Model file for the job. Use its own axes, mm. Round coordinates to 2 decimals unless told otherwise and drop trailing zeros. Order: outer loops, then holes, each group sorted by start corner. A loop starts at its lowest first (then second) coordinate and runs counter-clockwise, first axis right, second up. Notation, with made-up numbers: (-9.5, -19) - (-5.5, -19) arc R22 ccw to (-5.5, -11) - close; hole circle Ø3 at (45.5, 11). An arc over 180 degrees is marked (long way). Put each result on its own line as item: value. Start each with the question number.
Item 1: Mould opens along Z. For faces 1 (the face through (-0.29, 1.68, -1.32)), 2 (the face through (-2, 0, 0)), 3 (the face through (0.867, 0.197, 3.905)) say: pulls with the +Z half, pulls with the -Z half, needs draft (parallel to the pull), parting line crosses it, or undercut.
Item 2: Saw through at B-B on x = 0. List the corners of the cut face in (y, z), plus the area to 3 significant figures.
Item 3: Probe probe 1 along Z at (x, y) = (0, 2.5); probe 2 along Y at (x, z) = (3.25, -1.75); probe 3 along Z at (x, y) = (-1, 2.9). List the from-to ranges inside material, lowest first.
Item 4: Saw through at D-D on x = 1.75. List the corners of the cut face in (y, z).
Item 5: Saw through at C-C on z = -2.5. List the corners of the cut face in (x, y).
Item 6: Saw through at A-A on z = 0. List the corners of the cut face in (x, y).
Item 7: Pin check, flat tips, straight feed: pin 1 Ø2 at (x, y) = (-2, 1) entering from -Z; pin 2 Ø2 at (x, y) = (-2, 0.5) entering from -Z; pin 3 Ø1.5 at (x, y) = (3, 3) entering from +Z. Stop position of each tip, or through.
Autodesk Inventor part; units mm, degrees
ref_plane "YZ Plane" through (0, 0, 0) normal (1, 0, 0) x (0, 1, 0)
ref_plane "XZ Plane" through (0, 0, 0) normal (0, 1, 0) x (-1, 0, 0)
ref_plane "XY Plane" through (0, 0, 0) normal (0, 0, 1) x (1, 0, 0)
sketch "スケッチ1" plane through (0, 0, 0) normal (0, 1, 0) x (-1, 0, 0)
  circle A0 centre (0, 0) radius 4
  dimension "d0" = 8
extrude "押し出し1" add sketch "スケッチ1" along normal blind 0.4
sketch "スケッチ2" plane through (0, 0.4, 0) normal (0, 1, 0) x (1, 0, 0)
  circle A0 centre (0, 0) radius 3
  dimension "d3" = 6
extrude "押し出し2" add sketch "スケッチ2" along normal blind 3
sketch "スケッチ3" plane through (0, 0, 0) normal (0, -1, 0) x (1, 0, 0)
  circle A0 centre (0, 0) radius 1.35
  dimension "d6" = 2.7
extrude "押し出し3" cut sketch "スケッチ3" against normal through all
properties part number "screw_bearing_setter"
Results found:
1. face 1: undercut
1. face 2: needs draft
1. face 3: parting line crosses it
2. outline: (0, -4) - (0.4, -4) - (0.4, -3) - (3.4, -3) - (3.4, -1.35) - (0, -1.35) - close; (0, 1.35) - (3.4, 1.35) - (3.4, 3) - (0.4, 3) - (0.4, 4) - (0, 4) - close
2. area: 12.0 mm²
3. probe 1: z = -3 to -1.35, 1.35 to 3
3. probe 2: y = 0 to 0.4
3. probe 3: z = -2.83 to -0.91, 0.91 to 2.83
4. outline: (0, -3.6) - (0.4, -3.6) - (0.4, -2.44) - (3.4, -2.44) - (3.4, 2.44) - (0.4, 2.44) - (0.4, 3.6) - (0, 3.6) - close
5. outline: (-3.12, 0) - (3.12, 0) - (3.12, 0.4) - (1.66, 0.4) - (1.66, 3.4) - (-1.66, 3.4) - (-1.66, 0.4) - (-3.12, 0.4) - close
6. outline: (-4, 0) - (-1.35, 0) - (-1.35, 3.4) - (-3, 3.4) - (-3, 0.4) - (-4, 0.4) - close; (1.35, 0) - (4, 0) - (4, 0.4) - (3, 0.4) - (3, 3.4) - (1.35, 3.4) - close
7. pin 1: stops at z = -3.82
7. pin 2: stops at z = -3.87
7. pin 3: stops at z = 1.98
